```python
from build123d import *

# Parameters (mm, degrees)
SKETCH_W      = 54.7
SKETCH_H      = 127
PAD_DEPTH     = 5
SKETCH001_R   = 2.15
SKETCH001_R_2 = 22.5
PAD001_DEPTH  = 5
SKETCH002_R   = 2.15
SKETCH002_R_2 = 22.5
POCKET_DEPTH  = 3


with BuildPart() as part:
    # Sketch → Pad (new body)
    with BuildSketch(Plane.XY):
        with Locations((27.35, 63.5)):
            Rectangle(SKETCH_W, SKETCH_H)
    extrude(amount=-PAD_DEPTH)

    # Sketch001 → Pad001 (join)
    with BuildSketch(Plane.XY):
        Polygon((2.8, 2.8), (51.9, 2.8), (51.9, 74.2), (51.9, 124.2), (2.8, 124.2), (2.8, 74.2), align=None)
        with Locations((27.35, 12.823933)):
            Circle(SKETCH001_R, mode=Mode.SUBTRACT)
        with Locations((27.35, 64.223933)):
            Circle(SKETCH001_R, mode=Mode.SUBTRACT)
        with Locations((27.35, 38.523933)):
            Circle(SKETCH001_R_2, mode=Mode.SUBTRACT)
    extrude(amount=PAD001_DEPTH)

    # Sketch002 → Pocket (cut)
    with BuildSketch(Plane.XY):
        with Locations((27.35, 12.823933)):
            Circle(SKETCH002_R)
        with Locations((27.35, 64.223933)):
            Circle(SKETCH002_R)
        with Locations((27.35, 38.523933)):
            Circle(SKETCH002_R_2)
    extrude(amount=-POCKET_DEPTH, mode=Mode.SUBTRACT)


solid = part.part
```
Design review of the part built by this model. Coordinates are the model's own, in mm. A direction names the side the tool comes from. Give positions to 0.01 mm unless a question says otherwise; leave off trailing zeros. Order: outer loops, then holes, each group sorted by start corner. A loop starts at its lowest first (then second) coordinate and runs counter-clockwise, first axis right, second up. Notation, with made-up numbers: (-18, -8) - (34, -8) arc R21 cw to (34, 21) - close; hole circle Ø1 at (22.25, -26.5). An arc over 180 degrees is marked (long way). Use a Markdown table: item, result. Add a question column.
(1) Machinability: for faces 1 (the face through (29.4, 13.47, 0.94)), 2 (the face through (28, 124.2, 2)), 3 (the face through (27, 2.8, 2)), 4 (the face through (54.7, 63, -2)), 5 (the face through (2.8, 64, 2)), which of the approach directions +Z, -Z, +X, -X, +Y, -Y give a long, thin tool a straight path to every point of the face, cutting with its end or side? Answer none if there is none.
(2) Add section D-D on y = 18. Give the boundary of the cut face in (x, z).
(3) Mouldability with a two-part tool opening along X and no side actions: class faces 6 (the face through (27, 13, -3)), 7 (the face through (51.9, 63, 2)), 8 (the face through (27, 0, -2)) as +X half, -X half, draft (parallel to the pull), parting line (faces both ways), or undercut.
(4) Add section B-B on z = -1.75. Give the boundary of the cut face in (x, y), then the cut area to 3 significant figures.
(5) Add section A-A on y = 77.5. Give the boundary of the cut face in (x, z).
(6) Wall thickness on probe 1 along Y at (x, z) = (27.35, 2.5); probe 2 along Y at (x, z) = (4, 1.25); probe 3 along X at (y, z) = (37.5, 1.75): over which ranges is each line inside the solid? List them lowest first. Write a range as [from, to].
(7) Clearance check with flat-ended pins moving along their axes: P1, Ø5.5, axis at y = 92, z = 3.5, coming from the +X side; P2, Ø3.5, axis at x = 27.35, y = 64.22, coming from the +Z side; P3, Ø6, axis at x = 34, z = 3.5, coming from the +Y side. State where each tip first meets the part, or that it passes through.
(8) Add section C-C on x = 27.35. Give the boundary of the cut face in (y, z), then the cut area to 3 significant figures.
Report:
| question | item | result |
|---|---|---|
| 1 | face 1 | +Z |
| 1 | face 2 | +Z, +X, -X, +Y |
| 1 | face 3 | +Z, +X, -X, -Y |
| 1 | face 4 | +Z, -Z, +X, +Y, -Y |
| 1 | face 5 | +Z, -X, +Y, -Y |
| 2 | outline | (0, -5) - (54.7, -5) - (54.7, 0) - (51.9, 0) - (51.9, 5) - (36.57, 5) - (36.57, -3) - (18.13, -3) - (18.13, 5) - (2.8, 5) - (2.8, 0) - (0, 0) - close |
| 3 | face 6 | undercut |
| 3 | face 7 | +X half |
| 3 | face 8 | draft |
| 4 | outline | (0, 0) - (54.7, 0) - (54.7, 127) - (0, 127) - close; hole circle Ø45 at (27.35, 38.52); hole circle Ø4.3 at (27.35, 12.82); hole circle Ø4.3 at (27.35, 64.22) |
| 4 | area | 5,330 mm² |
| 5 | outline | (0, -5) - (54.7, -5) - (54.7, 0) - (51.9, 0) - (51.9, 5) - (2.8, 5) - (2.8, 0) - (0, 0) - close |
| 6 | probe 1 | y = [2.8, 10.67], [14.97, 16.02], [61.02, 62.07], [66.37, 124.2] |
| 6 | probe 2 | y = [2.8, 124.2] |
| 6 | probe 3 | x = [2.8, 4.87], [49.83, 51.9] |
| 7 | P1 | stops at x = 51.9 |
| 7 | P2 | stops at z = -3 |
| 7 | P3 | stops at y = 124.2 |
| 8 | outline | (0, -5) - (127, -5) - (127, 0) - (124.2, 0) - (124.2, 5) - (66.37, 5) - (66.37, -3) - (62.07, -3) - (62.07, 5) - (61.02, 5) - (61.02, -3) - (16.02, -3) - (16.02, 5) - (14.97, 5) - (14.97, -3) - (10.67, -3) - (10.67, 5) - (2.8, 5) - (2.8, 0) - (0, 0) - close |
| 8 | area | 813 mm² |
